```python
from build123d import *

# Parameters (mm, degrees)
SKETCH1_R                = 2.150000002
SKETCH1_R_2              = 35
SKETCH1_R_3              = 1.8
SKETCH1_R_4              = 7.575
BOSS_EXTRUDE1_DEPTH      = 3.175
SKETCH3_R                = 1.35
SKETCH3_R_2              = 5
SKETCH3_W                = 18
SKETCH3_H                = 3.5
CUT_EXTRUDE1_DEPTH       = 3.175
CUT_EXTRUDE2_DEPTH       = 3.175
SKETCH6_R                = 7.5
CUT_EXTRUDE5_DEPTH       = 10
FILLET1_R                = 1.75
SKETCH7_R                = 1.75
CUT_EXTRUDE6_DEPTH       = 10
SKETCH10_R               = 1.8
BOSS_EXTRUDE2_DEPTH      = 2.3
CUT_EXTRUDE7_DEPTH       = 118.49445714
CUT_EXTRUDE7_DEPTH_BACK  = 118.49445714
SKETCH11_W               = 179.014242855
SKETCH11_H               = 40.200555742
BOSS_EXTRUDE3_DEPTH      = 9.5
BOSS_EXTRUDE3_DEPTH_BACK = 2.3
CHAMFER1_SIZE            = 0.5


with BuildPart() as part:
    # Sketch1 → Boss-Extrude1 (new body)
    with BuildSketch(Plane.XY):
        with BuildLine():
            Line((69.097259206, -18.820036388), (54.057762213, -10.136978751))
            ThreePointArc((54.057762213, -10.136978751), (47.631397163, 27.499999965), (18.250000006, 51.883884719))
            Line((18.250000006, 51.883884719), (18.250000006, 69.249999994))
            ThreePointArc((18.250000006, 69.249999994), (6e-09, 87.499999994), (-18.249999994, 69.249999994))
            Line((-18.249999994, 69.249999994), (-18.249999994, 51.883884717))
            ThreePointArc((-18.249999994, 51.883884717), (-47.836716311, 27.141270525), (-53.899300523, -10.948305635))
            Line((-53.899300523, -10.948305635), (-69.097259204, -18.820036383))
            ThreePointArc((-69.097259204, -18.820036383), (-77.600405532, -29.901552426), (-75.777222821, -43.749999994))
            ThreePointArc((-75.777222821, -43.749999994), (0, -87.499999989), (75.777222821, -43.749999994))
            ThreePointArc((75.777222821, -43.749999994), (77.60040553, -29.901552429), (69.097259206, -18.820036388))
        make_face()
        with Locations((-7.778174593, 77.028174587)):
            Circle(SKETCH1_R, mode=Mode.SUBTRACT)
        Circle(SKETCH1_R_2, mode=Mode.SUBTRACT)
        with Locations((-50, 0)):
            Circle(SKETCH1_R_3, mode=Mode.SUBTRACT)
        with Locations((-25, 43.301270189)):
            Circle(SKETCH1_R_3, mode=Mode.SUBTRACT)
        with Locations((25, 43.301270189)):
            Circle(SKETCH1_R_3, mode=Mode.SUBTRACT)
        with Locations((50, 0)):
            Circle(SKETCH1_R_3, mode=Mode.SUBTRACT)
        with Locations((25, -43.301270189)):
            Circle(SKETCH1_R_3, mode=Mode.SUBTRACT)
        with Locations((-25, -43.301270189)):
            Circle(SKETCH1_R_3, mode=Mode.SUBTRACT)
        with Locations((7.778174587, 77.028174593)):
            Circle(SKETCH1_R, mode=Mode.SUBTRACT)
        with Locations((7.778174593, 61.471825413)):
            Circle(SKETCH1_R, mode=Mode.SUBTRACT)
        with Locations((-7.778174587, 61.471825407)):
            Circle(SKETCH1_R, mode=Mode.SUBTRACT)
        with Locations((62.819268711, -45.250184084)):
            Circle(SKETCH1_R, mode=Mode.SUBTRACT)
        with Locations((49.347075128, -37.472009499)):
            Circle(SKETCH1_R, mode=Mode.SUBTRACT)
        with Locations((57.125249713, -23.999815916)):
            Circle(SKETCH1_R, mode=Mode.SUBTRACT)
        with Locations((70.597443296, -31.777990501)):
            Circle(SKETCH1_R, mode=Mode.SUBTRACT)
        with Locations((-70.597443298, -31.777990509)):
            Circle(SKETCH1_R, mode=Mode.SUBTRACT)
        with Locations((-57.125249721, -23.999815914)):
            Circle(SKETCH1_R, mode=Mode.SUBTRACT)
        with Locations((-49.347075126, -37.472009491)):
            Circle(SKETCH1_R, mode=Mode.SUBTRACT)
        with Locations((-62.819268703, -45.250184086)):
            Circle(SKETCH1_R, mode=Mode.SUBTRACT)
        with Locations((0, 69.249999994)):
            Circle(SKETCH1_R_4, mode=Mode.SUBTRACT)
        with Locations((59.972259207, -34.624999997)):
            Circle(SKETCH1_R_4, mode=Mode.SUBTRACT)
        with Locations((-59.972259207, -34.624999997)):
            Circle(SKETCH1_R_4, mode=Mode.SUBTRACT)
    extrude(amount=BOSS_EXTRUDE1_DEPTH)

    # Sketch3 → Cut-Extrude1 (cut)
    with BuildSketch(Plane.XY.offset(3.175)):
        with Locations((-33.85, -49)):
            Circle(SKETCH3_R)
        with Locations((-33.85, -75)):
            Circle(SKETCH3_R)
        with Locations((41.45, -46.7)):
            Circle(SKETCH3_R)
        with Locations((49.972259207, -51.945508073)):
            Circle(SKETCH3_R_2)
        with Locations((48.55, -69)):
            Circle(SKETCH3_R)
        with Locations((30, -36.05)):
            Rectangle(SKETCH3_W, SKETCH3_H)
    extrude(amount=-CUT_EXTRUDE1_DEPTH, mode=Mode.SUBTRACT)

    # Sketch4 → Cut-Extrude2 (cut)
    with BuildSketch(Plane.XY.offset(3.175)):
        Polygon((-18.902035191, 65.231994187), (-24.642286676, 79.090187175), (-38.500479664, 73.349935689), (-32.760228178, 59.491742702), align=None)
        Polygon((-47.04154651, -48.985639752), (-56.172967945, -60.885939856), (-63.507557332, -70.444562845), (-51.607257228, -79.57598428), (-44.272667841, -70.017361292), (-35.141246406, -58.117061187), align=None)
        Polygon((65.943581701, -16.246354435), (80.815254622, -18.204247318), (82.773147505, -3.332574398), (67.901474584, -1.374681515), align=None)
    extrude(amount=-CUT_EXTRUDE2_DEPTH, mode=Mode.SUBTRACT)

    # Sketch6 → Cut-Extrude5 (cut)
    with BuildSketch(Plane.XY):
        with Locations((20, 69.25)):
            Circle(SKETCH6_R)
        with Locations((-69.972259212, -17.304491924)):
            Circle(SKETCH6_R)
    extrude(amount=CUT_EXTRUDE5_DEPTH, mode=Mode.SUBTRACT)

    # Fillet1
    fillet1_edges = [part.edges().sort_by_distance(p)[0] for p in [
        (21, -37.8, 1.5875),
        (39, -37.8, 1.5875),
        (39, -34.3, 1.5875),
        (21, -34.3, 1.5875),
    ]]
    fillet(fillet1_edges, radius=FILLET1_R - 0.0001)  # a hair under: the kernel refuses the full size

    # Sketch7 → Cut-Extrude6 (cut)
    with BuildSketch(Plane.XY.offset(3.175)):
        with Locations((-43, 10)):
            Circle(SKETCH7_R)
        with Locations((-43, -10)):
            Circle(SKETCH7_R)
    extrude(amount=-CUT_EXTRUDE6_DEPTH, mode=Mode.SUBTRACT)

    # Sketch10 → Boss-Extrude2 (add)
    with BuildSketch(Plane.XY.offset(3.175)):
        with BuildLine():
            Line((29.492976073, -37.8), (37.25, -37.8))
            ThreePointArc((37.25, -37.8), (38.487436867, -37.287436867), (39, -36.05))
            ThreePointArc((39, -36.05), (38.487436867, -34.812563133), (37.25, -34.3))
            Line((37.25, -34.3), (29.492976073, -34.3))
            ThreePointArc((29.492976073, -34.3), (29.307916131, -33.656774505), (29.066247328, -33.032609135))
            ThreePointArc((29.066247328, -33.032609135), (42.625064482, -10.913472313), (41.36423576, 15))
            Line((41.36423576, 15), (52.915026221, 15))
            ThreePointArc((52.915026221, 15), (52.809487392, -15.367434443), (36.604610365, -41.05))
            Line((36.604610365, -41.05), (27.790169944, -41.05))
            ThreePointArc((27.790169944, -41.05), (28.843379247, -39.530734431), (29.492976073, -37.8))
        make_face()
        with Locations((50, 0)):
            Circle(SKETCH10_R, mode=Mode.SUBTRACT)
    extrude(amount=BOSS_EXTRUDE2_DEPTH)

    # Sketch11 → Cut-Extrude7 (cut, two sides: drawn at the far end of the back side and taken through both)
    with BuildSketch(Plane(origin=(0, 0, 0), x_dir=(1, 0, 0), z_dir=(0, 1, 0)).offset(-CUT_EXTRUDE7_DEPTH_BACK)):
        with Locations((-6.278377224, 16.925277871)):
            Rectangle(SKETCH11_W, SKETCH11_H)
    extrude(amount=CUT_EXTRUDE7_DEPTH + CUT_EXTRUDE7_DEPTH_BACK, mode=Mode.SUBTRACT)

    # Sketch12 → Boss-Extrude3 (add, two sides: drawn at the far end of the back side and taken through both)
    with BuildSketch(Plane(origin=(0, 0, 3.175), x_dir=(-1, 0, 0), z_dir=(0, 0, -1)).offset(-BOSS_EXTRUDE3_DEPTH_BACK)):
        with BuildLine():
            Line((-29.492976073, -37.8), (-37.25, -37.8))
            ThreePointArc((-37.25, -37.8), (-38.487436867, -37.287436867), (-39, -36.05))
            ThreePointArc((-39, -36.05), (-38.487436867, -34.812563133), (-37.25, -34.3))
            Line((-37.25, -34.3), (-29.492976073, -34.3))
            ThreePointArc((-29.492976073, -34.3), (-29.7, -36.05), (-29.492976073, -37.8))
        make_face()
    extrude(amount=BOSS_EXTRUDE3_DEPTH + BOSS_EXTRUDE3_DEPTH_BACK)

    # Chamfer1
    chamfer1_edges = [part.edges().sort_by_distance(p)[0] for p in [
        (29.7, -36.05, -6.325),
        (33.371488036, -34.3, -6.325),
        (39, -36.05, -6.325),
        (33.371488036, -37.8, -6.325),
    ]]
    chamfer(chamfer1_edges, length=CHAMFER1_SIZE)


solid = part.part
```
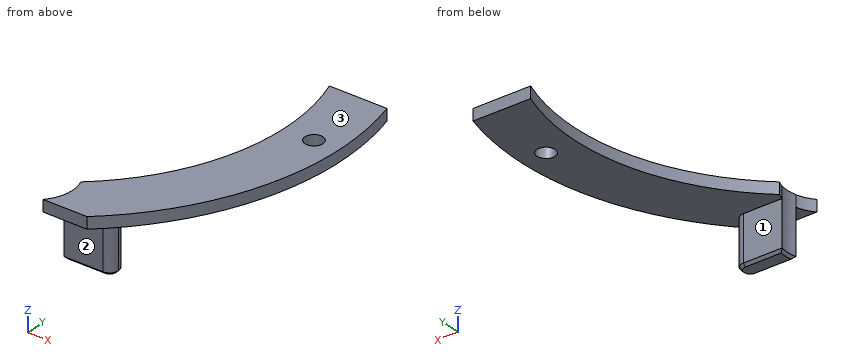
Check sheet for the modelled part. Datum: model origin and axes. Units: mm. Face numbers are marked on the shaded views. A direction names the side the tool comes from. Coordinates: 2 decimals unless noted, no trailing zeros. Loops run counter-clockwise (first coordinate to the right, second up) from the corner with the lowest first, then second, coordinate; pieces in that order, holes last. Notation, with made-up numbers: M 3.25,18 L 36.25,18 A14 ccw 36.25,26 Z; hole C -22.5,49.25 d1. An arc over 180 degrees is marked long. Answer as a JSON object with one key per item and string values.
1. Sectioned sample at A-A on y = 0. Record the cut outline in (x, z) (3 decimals).
Outcome:
{"outline": "M 44,3.175 L 48.2,3.175 L 48.2,5.475 L 44,5.475 Z; M 51.8,3.175 L 55,3.175 L 55,5.475 L 51.8,5.475 Z"}
2. Sectioned sample at D-D on z = 0.5. Record the cut outline in (x, y).
Outcome:
{"outline": "M 29.49,-37.8 L 37.25,-37.8 A1.75 ccw 37.25,-34.3 L 29.49,-34.3 A7.5 cw Z"}
3. Sectioned sample at B-B on x = 50. Record the cut outline in (y, z) (3 decimals), and give its area (3 significant figures).
Outcome:
{"outline": "M -22.913,3.175 L -1.8,3.175 L -1.8,5.475 L -22.913,5.475 Z; M 1.8,3.175 L 15,3.175 L 15,5.475 L 1.8,5.475 Z", "area": "78.9 mm²"}
4. Access from +Z, -Z, +X, -X, +Y, -Y to the whole of each face (thin tool, end or side, straight path). Record for the marked faces 1, 2 and 3.
Outcome:
{"face 1": "-Z, +X, -X, +Y", "face 2": "-Z, +X, -X, -Y", "face 3": "+Z, +X, -X, +Y, -Y"}
5. Sectioned sample at C-C on z = 3.75. Record the cut outline in (x, y).
Outcome:
{"outline": "M 27.79,-41.05 L 36.6,-41.05 A55 ccw 52.92,15 L 41.36,15 A44 cw 29.07,-33.03 A7.5 cw Z; hole C 50,0 d3.6"}
6. Depth check by flat-ended pin: P1, Ø5, axis at y = -10.5, z = 4, coming from the -X side; P2, Ø10, axis at x = 43.5, y = -23.5, coming from the -Z side (3 decimals); P3, Ø2.5, axis at x = 33.5, z = -0.5, coming from the +Y side. Enter the tip coordinate at first touch or a pass-through.
Outcome:
{"P1": "x = 42.04", "P2": "z = 3.175", "P3": "y = -34.3"}
7. Scan lines: L1, parallel to X at y = 0, z = 4.2; L2, parallel to Z at x = 48.25, y = 9 (3 decimals); L3, parallel to Y at x = 50, z = 4.55. Record each from-to range of solid material in increasing order. Write a range as from..to.
Outcome:
{"L1": "44..48.2, 51.8..55", "L2": "3.175..5.475", "L3": "-22.91..-1.8, 1.8..15"}
